Read the model definition and answer for the solid it produces. Units are mm, in the model's axes. A direction names the side the tool comes from. Coordinates: 2 decimals unless noted, no trailing zeros. Order: outer loops, then holes, each group sorted by start corner. A loop starts at its lowest first (then second) coordinate and runs counter-clockwise, first axis right, second up. Notation, with made-up numbers: M -26,80.5 L 8,80.5 A10 ccw 8,91.5 Z; hole C -20.75,64 d4. An arc over 180 degrees is marked long. Put each result on its own line as item: value.
Solid Edge part; units mm, degrees
sketch "Sketch1" plane through (0, 0, 0) normal (0, -1, 0) x (1, 0, 0)
  line L0 (-168.6518, -24.5) -> (-39.896, 10)
  line L1 (-39.896, 10) -> (30.104, 10)
  arc A0 (30.104, 10) -> (30.104, -10) centre (30.104, 0) cw
  line L2 (30.104, -10) -> (-39.896, -10)
  line L3 (-39.896, -10) -> (-39.896, -34.5)
  line L4 (-39.896, -34.5) -> (-168.6518, -34.5)
  line L5 (-168.6518, -34.5) -> (-168.6518, -24.5)
  circle A1 centre (30.104, 0) radius 5
  circle A2 centre (0, 0) radius 5
  dimension "D1" = 39.896
  dimension "D2" = 39.896
  dimension "D3" = 168.6518
  dimension "D4" = 39.896
extrude "Protrusion1" add sketch "Sketch1" along normal mid plane 4
sketch "Sketch2" plane through (-34.896, 0, -4.3782) normal (0, -1, 0) x (1, 0, 0)
  line L0 (-5, -5.6218) -> (-133.7558, -5.6218)
  line L1 (-133.7558, -19.3921) -> (-133.7558, -5.6218)
  line L2 (-131.6787, -19.5652) -> (-133.7558, -19.3921)
  line L3 (-5, -30.1218) -> (-131.6787, -19.5652)
  line L4 (-5, -5.6218) -> (-5, -30.1218)
  dimension "D1" = 5
extrude "Protrusion2" add sketch "Sketch2" along normal mid plane 15
fillet "Redondeo_2" radius 3 1 edges at (-39.896, 0, -10)
sketch "Sketch3" plane through (-74.896, -7.5, -22.0833) normal (0.9965458, 0, -0.0830455) x (0, 1, 0)
  line L0 (7.5, -4.4672) -> (2.5, -9.4672)
  line L1 (2.5, -9.4672) -> (12.5, -9.4672)
  line L2 (7.5, -4.4672) -> (12.5, -9.4672)
  dimension "D1" = 7.5
extrude "Cutout1" cut sketch "Sketch3" along normal through all and the other way through all
sketch "Sketch4" plane through (-104.2739, -2, -29.2217) normal (0, -1, 0) x (1, 0, 0)
  line L0 (-64.3779, 5.4514) -> (64.3779, -5.2783)
  line L1 (64.3779, -5.2783) -> (-64.3779, -5.2783)
  line L2 (-64.3779, -5.2783) -> (-64.3779, 5.4514)
extrude "Cutout2" cut sketch "Sketch4" along normal through all and the other way through all
Q1. A tool of negligible diameter and unlimited length cuts with its end or side. For faces 1 (the face through (40.1, 0, 0.2)), 2 (the face through (-103, 3, -10)), 3 (the face through (-3, 0, -10)), 4 (the face through (-105.18, -2.47, -26.52)), 5 (the face through (-77.74, 0.03, -0.14)), from which of +Z, -Z, +X, -X, +Y, -Y can it reach the whole face along a straight path? Write none if from no direction.
Answers below:
face 1: +X, +Y, -Y
face 2: +Z, -X
face 3: -Z, +X, +Y, -Y
face 4: -Z, -X
face 5: +Z, -X, +Y, -Y
Q2. Find section A-A on x = 0. Write down the section's boundary in (y, z), plus the area to 3 significant figures.
Answers below:
outline: M -2,-10 L 2,-10 L 2,-5 L -2,-5 Z; M -2,5 L 2,5 L 2,10 L -2,10 Z
area: 40.0 mm^2
Q3. For a pull along Z with two mould halves and no side action, classify faces 6 (the face through (-39.896, 0, -22)), 7 (the face through (-1.08, 0.03, 4.88)), 8 (the face through (-5, 0, 10)) as +Z half, -Z half, draft (parallel to the pull), parting line (faces both ways), or undercut.
Answers below:
face 6: draft
face 7: undercut
face 8: +Z half
Q4. Given pin 1 (6 mm diameter, centred on x = 0, z = 0, fed in from +Y); pin 2 (3 mm diameter, centred on x = -3.5, y = 1, fed in from -Z); pin 3 (7 mm diameter, centred on x = -31.5, z = 4, fed in from +Y); pin 4 (2 mm diameter, centred on x = -114, y = 0, fed in from +Z), each flat-ended and moving along its own axis, determine where each tip first touches the part or whether it passes through.
Answers below:
pin 1: passes through
pin 2: stops at z = -10
pin 3: stops at y = 2
pin 4: stops at z = -9.59
Q5. Find section D-D on x = -49.5. Write down the section's boundary in (y, z), plus the area to 3 significant figures.
Answers below:
outline: M -7.5,-33.7 L -5,-33.7 L 0,-28.68 L 5,-33.7 L 7.5,-33.7 L 7.5,-10 L 2,-10 L 2,7.43 L -2,7.43 L -2,-10 L -7.5,-10 Z
area: 400 mm^2
Q6. Find section C-C on x = -129.5. Write down the section's boundary in (y, z), plus the area to 3 significant figures.
Answers below:
outline: M -7.5,-27.03 L -5,-27.03 L 0,-22.02 L 5,-27.03 L 7.5,-27.03 L 7.5,-10 L -7.5,-10 Z
area: 230 mm^2
Q7. Find section B-B on z = 0. Write down the section's boundary in (x, y).
Answers below:
outline: M -77.22,-2 L -5,-2 L -5,2 L -77.22,2 Z; M 5,-2 L 25.1,-2 L 25.1,2 L 5,2 Z; M 35.1,-2 L 40.1,-2 L 40.1,2 L 35.1,2 Z
Q8. Consider line 1 along Z through (x, y) = (-36.5, 1.75); line 2 along X through (y, z) = (-2, -18.5); line 3 along Y through (x, z) = (-42, 1). Determine where each line is inside the solid, lowest interval first.
Answers below:
line 1: z = -10 to 10
line 2: x = -168.65 to -39.9
line 3: y = -2 to 2
